from build123d import *

# Parameters (mm, degrees)
F0_R     = 30
F1_DEPTH = 4.2
F2_R     = 8.5
F2_R_2   = 8
F3_DEPTH = 10


with BuildPart() as f1:
    # F0 (on Front) → F1 (new body)
    with BuildSketch(Plane.XZ):
        Circle(F0_R)
    extrude(amount=F1_DEPTH)

    # F2 (on face) → F3 (join)
    with BuildSketch(Plane.XZ.offset(4.2)):
        Circle(F2_R)
        Circle(F2_R_2, mode=Mode.SUBTRACT)
    extrude(amount=F3_DEPTH)

    # F4 (on Top) → F5 (revolve, cut)
    with BuildSketch(Plane.XY):
        Polygon((28.669611, -2.787452), (30.564366, -4.003254), (30.564366, -0.213743), (28.669611, -1.310707), align=None)
    revolve(axis=Axis((0, -2.633361, 0), (0, -1, 0)), mode=Mode.SUBTRACT)


solid = f1.part
Verification items for the finished model (mm, model axes). A direction names the side the tool comes from. Round coordinates to 2 decimals unless told otherwise and drop trailing zeros. Loops run counter-clockwise (first coordinate to the right, second up) from the corner with the lowest first, then second, coordinate; pieces in that order, holes last. Notation, with made-up numbers: (7.5, -24) - (51.5, -24) arc R24 cw to (51.5, -3) - close; hole circle Ø10 at (89, -33). An arc over 180 degrees is marked (long way). Use one line per item in the form item = value.
1. Draft check along Y on faces 1 (the cylindrical face through (-29.97, -0.27, 1.32)), 2 (the flat face through (0, 0, 0)), 3 (the cylindrical face through (26.483, -2.059, -10.981)). Enter one of: pulls with the +Y half, pulls with the -Y half, needs draft (parallel to the pull), parting line crosses it, or undercut.
A:
face_1 = needs draft
face_2 = pulls with the +Y half
face_3 = undercut
2. Section check A-A on x = 0. Record the cut outline in (y, z).
A:
outline = (-14.2, -8.5) - (-4.2, -8.5) - (-4.2, -30) - (-3.64, -30) - (-2.79, -28.67) - (-1.31, -28.67) - (-0.54, -30) - (0, -30) - (0, 30) - (-0.54, 30) - (-1.31, 28.67) - (-2.79, 28.67) - (-3.64, 30) - (-4.2, 30) - (-4.2, 8.5) - (-14.2, 8.5) - (-14.2, 8) - (-4.2, 8) - (-4.2, -8) - (-14.2, -8) - close
3. Access from +Z, -Z, +X, -X, +Y, -Y to the whole of each face (thin tool, end or side, straight path). Record for faces 4 (the cylindrical face through (-29.97, -3.92, 1.32)), 5 (the flat face through (0, -4.2, 0)).
A:
face_4 = +Y, -Y
face_5 = -Y
4. Scan lines: probe 1 along Z at (x, y) = (0, -8); probe 2 along Y at (x, z) = (8, -6.5); probe 3 along X at (y, z) = (-6, 4). Record each from-to range of solid material in increasing order.
A:
probe_1 = -8.5 to -8, 8 to 8.5
probe_2 = -4.2 to 0
probe_3 = -7.5 to -6.93, 6.93 to 7.5
5. Section check C-C on y = -6.25. Record the cut outline in (x, z), and give its area (3 significant figures).
A:
outline = circle Ø17 at (0, 0); hole circle Ø16 at (0, 0)
area = 25.9 mm²
6. Gauge pin test, flat ends, axial feed: pin 1 Ø3 at (y, z) = (-4.5, 8) entering from +X; pin 2 Ø8 at (x, z) = (-20, 2) entering from +Y; pin 3 Ø1.5 at (x, y) = (-7.5, -4) entering from +Z; pin 4 Ø1.5 at (x, z) = (-21, -12.5) entering from -Y. Record the tip position at first contact, or that the pin passes through.
A:
pin_1 = 29.28
pin_2 = 0
pin_3 = 29.23
pin_4 = -4.2
7. Section check B-B on z = 0. Record the cut outline in (x, y), and give its area (3 significant figures).
A:
outline = (-30, -4.2) - (-8.5, -4.2) - (-8.5, -14.2) - (-8, -14.2) - (-8, -4.2) - (8, -4.2) - (8, -14.2) - (8.5, -14.2) - (8.5, -4.2) - (30, -4.2) - (30, -3.64) - (28.67, -2.79) - (28.67, -1.31) - (30, -0.54) - (30, 0) - (-30, 0) - (-30, -0.54) - (-28.67, -1.31) - (-28.67, -2.79) - (-30, -3.64) - close
area = 256 mm²
8. Section check D-D on y = -2. Record the cut outline in (x, z).
A:
outline = circle Ø57.34 at (0, 0)
